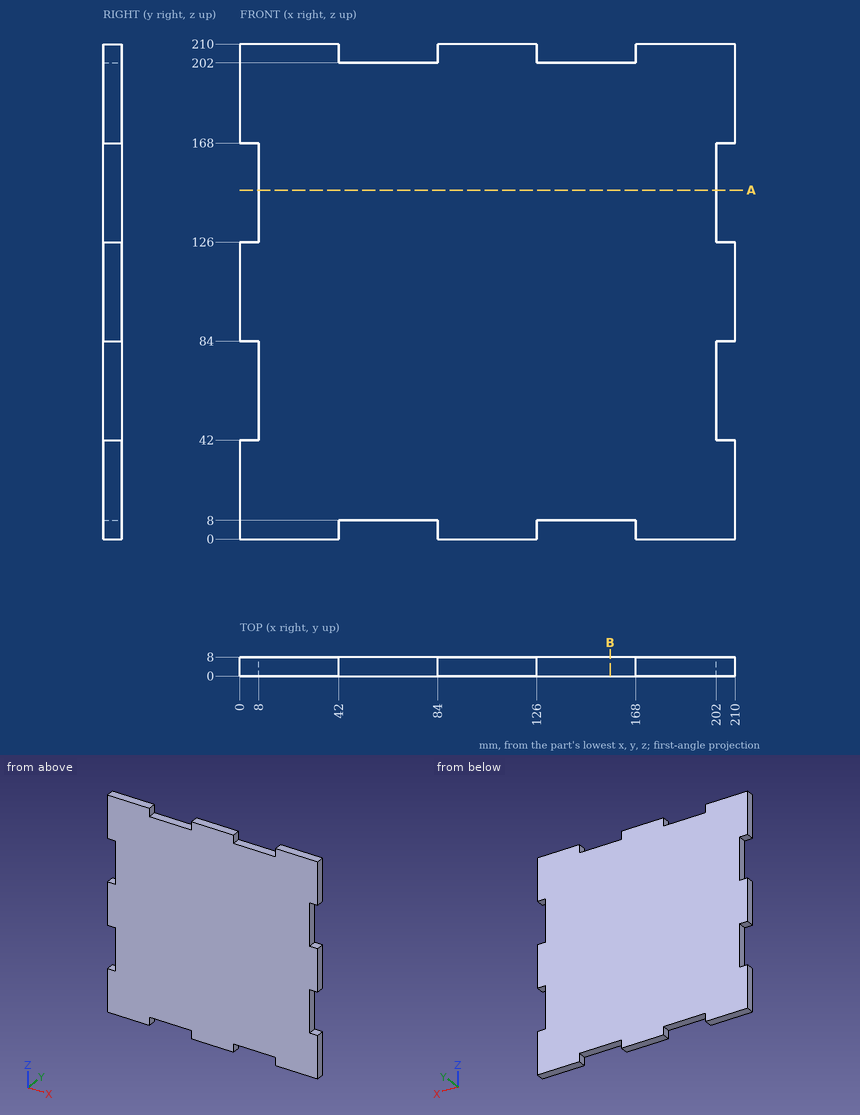
Drawing for the job (mm, zero at the part's lowest x, y, z). Round coordinates to 2 decimals unless told otherwise and drop trailing zeros. Loops run counter-clockwise (first coordinate to the right, second up) from the corner with the lowest first, then second, coordinate; pieces in that order, holes last. Notation, with made-up numbers: (48, -19.75) -> (65, -19.75) arc R18 cw to (65, -3.75) -> close; hole circle Ø3 at (12.5, 40.5). An arc over 180 degrees is marked (long way). Answer as CSV lines item,"result". Start each with the question number.
1) Slice it at A-A (z = 148). List the corners of the cut face in (x, y), plus the area to 3 significant figures.
2) Slice it at B-B (x = 157). List the corners of the cut face in (y, z), plus the area to 3 significant figures.
3) Pin check, flat tips, straight feed: P1, Ø4, axis at x = 55, y = 5, coming from the -Z side; P2, Ø3, axis at y = 6, z = 80, coming from the +X side; P3, Ø1.5, axis at x = 131, z = 150, coming from the -Y side. Stop position of each tip, or through.
4) Probe line 1 along X through (y, z) = (3, 83.5). List the from-to ranges inside material, lowest first.
Filled in:
1,outline,"(8, 0) -> (202, 0) -> (202, 8) -> (8, 8) -> close"
1,area,"1,550 mm2"
2,outline,"(0, 8) -> (8, 8) -> (8, 202) -> (0, 202) -> close"
2,area,"1,550 mm2"
3,P1,"stops at z = 8"
3,P2,"stops at x = 202"
3,P3,"stops at y = 0"
4,line 1,"x = 8 to 202"
